```python
from build123d import *

# Parameters (mm, degrees)
F0_W     = 76.2
F0_H     = 63.5
F0_W_2   = 2.54
F0_H_2   = 27.94
F0_H_3   = 12.7
F1_DEPTH = 22.86
F2_W     = 76.2
F2_H     = 63.5
F3_DEPTH = 2.032
F4_R     = 1.27
F5_R     = 1


with BuildPart() as f1:
    # F0 (on Top) → F1 (new body)
    with BuildSketch(Plane.XY):
        with Locations((38.1, 31.75)):
            Rectangle(F0_W, F0_H)
        Polygon((2.54, 48.26), (2.54, 60.96), (73.66, 60.96), (73.66, 48.26), (73.66, 45.72), (73.66, 33.02), (73.66, 30.48), (73.66, 2.54), (41.4866666667, 2.54), (38.9466666667, 2.54), (22.0133333333, 2.54), (19.4733333333, 2.54), (2.54, 2.54), (2.54, 30.48), (2.54, 33.02), (2.54, 45.72), align=None, mode=Mode.SUBTRACT)
        Polygon((73.66, 48.26), (2.54, 48.26), (2.54, 45.72), (37.465, 45.72), (40.005, 45.72), (73.66, 45.72), align=None)
        Polygon((37.465, 33.02), (2.54, 33.02), (2.54, 30.48), (19.4733333333, 30.48), (22.0133333333, 30.48), (38.9466666667, 30.48), (41.4866666667, 30.48), (73.66, 30.48), (73.66, 33.02), (40.005, 33.02), align=None)
        with Locations((20.7433333333, 16.51)):
            Rectangle(F0_W_2, F0_H_2)
        with Locations((40.2166666667, 16.51)):
            Rectangle(F0_W_2, F0_H_2)
        with Locations((38.735, 39.37)):
            Rectangle(F0_W_2, F0_H_3)
    extrude(amount=F1_DEPTH)

    # F2 (on face) → F3 (join)
    with BuildSketch(Plane.XY.offset(22.86)):
        with Locations((38.1, 31.75)):
            Rectangle(F2_W, F2_H)
    extrude(amount=-F3_DEPTH)

    # F4
    f4_edges = [f1.edges().sort_by_distance(p)[0] for p in [
        (76.2, 31.75, 0),
        (38.1, 0, 0),
        (0, 31.75, 0),
        (38.1, 63.5, 0),
        (0, 63.5, 11.43),
        (76.2, 63.5, 11.43),
        (0, 0, 11.43),
        (76.2, 0, 11.43),
    ]]
    fillet(f4_edges, radius=F4_R)

    # F5
    f5_edges = [f1.edges().sort_by_distance(p)[0] for p in [
        (73.66, 60.96, 10.414),
        (73.66, 48.26, 10.414),
        (73.66, 33.02, 10.414),
        (73.66, 2.54, 10.414),
        (38.946667, 2.54, 10.414),
        (19.473333, 2.54, 10.414),
        (19.473333, 30.48, 10.414),
        (38.946667, 30.48, 10.414),
        (2.54, 30.48, 10.414),
        (2.54, 2.54, 10.414),
        (2.54, 45.72, 10.414),
        (2.54, 33.02, 10.414),
        (73.66, 45.72, 10.414),
        (41.486667, 30.48, 10.414),
        (41.486667, 2.54, 10.414),
        (2.54, 60.96, 10.414),
        (2.54, 48.26, 10.414),
        (73.66, 30.48, 10.414),
        (22.013333, 2.54, 10.414),
        (22.013333, 30.48, 10.414),
        (40.005, 33.02, 10.414),
        (40.005, 45.72, 10.414),
        (37.465, 45.72, 10.414),
        (37.465, 33.02, 10.414),
    ]]
    fillet(f5_edges, radius=F5_R)


solid = f1.part
```
Here's how the part is built. I have some questions about the finished solid (model axes, mm). A direction names the side the tool comes from. Round coordinates to 2 decimals unless told otherwise and drop trailing zeros. Loops run counter-clockwise (first coordinate to the right, second up) from the corner with the lowest first, then second, coordinate; pieces in that order, holes last. Notation, with made-up numbers: (-27.5, 8) -> (13.5, 8) arc R29 ccw to (13.5, 36) -> close; hole circle Ø8 at (84.5, 33). An arc over 180 degrees is marked (long way). Answer as CSV lines item,"result". Start each with the question number.
1. Imagine slicing it at D-D on y = 52.5. Write out the boundary of the cut face in (x, z).
2. If we mould it in two halves opening along Y, with no side actions, what happens to faces 1 (the face through (38, 0, 12)), 2 (the face through (20, 39, 20.828)), 3 (the face through (76.2, 31, 12)), 4 (the face through (11, 30.48, 10))? For each: pulls with the +Y half, pulls with the -Y half, needs draft (parallel to the pull), parting line crosses it, or undercut.
3. Imagine slicing it at B-B on x = 53.5. Write out the boundary of the cut face in (y, z), plus the area to 3 significant figures.
4. I'm going to push flat-ended pins straight in: P1, Ø10, axis at x = 21, y = 17.5, coming from the -Z side; P2, Ø4, axis at x = 49, y = 56.5, coming from the -Z side. Where does each tip first touch, or does it pass through?
5. Imagine slicing it at C-C on z = 10. State how many separate pieces and enclosed holes the cut face has, plus the area to 3 significant figures.
6. I need wall thicknesses on probe 1 along Y at (x, z) = (59, 17.5); probe 2 along X at (y, z) = (25.5, 10); probe 3 along X at (y, z) = (38.5, 8.5) (3 decimals). Which ranges of each line are inside material? Lowest first, please. Write a range as from..to.
7. For faces 5 (the face through (38, 32, 22.86)), 6 (the face through (57, 17, 20.828)), which set-ups out of +Z, -Z, +X, -X, +Y, -Y let a thin tool reach every point of the face, with its end or its side?
8. Imagine slicing it at A-A on y = 15.5. Write out the boundary of the cut face in (x, z).
Solution:
1,outline,"(0, 1.27) arc R1.27 ccw to (1.27, 0) -> (2.54, 0) -> (2.54, 20.83) -> (73.66, 20.83) -> (73.66, 0) -> (74.93, 0) arc R1.27 ccw to (76.2, 1.27) -> (76.2, 22.86) -> (0, 22.86) -> close"
2,face 1,"pulls with the -Y half"
2,face 2,"undercut"
2,face 3,"needs draft"
2,face 4,"undercut"
3,outline,"(0, 1.27) arc R1.27 ccw to (1.27, 0) -> (2.54, 0) -> (2.54, 20.83) -> (30.48, 20.83) -> (30.48, 0) -> (33.02, 0) -> (33.02, 20.83) -> (45.72, 20.83) -> (45.72, 0) -> (48.26, 0) -> (48.26, 20.83) -> (60.96, 20.83) -> (60.96, 0) -> (62.23, 0) arc R1.27 ccw to (63.5, 1.27) -> (63.5, 22.86) -> (0, 22.86) -> close"
3,area,"340 mm²"
4,P1,"z = 0"
4,P2,"z = 20.83"
5,separate pieces,"1"
5,enclosed holes,"6"
5,area,"1,220 mm²"
6,probe 1,"0..2.54, 30.48..33.02, 45.72..48.26, 60.96..63.5"
6,probe 2,"0..2.54, 19.47..22.01, 38.95..41.49, 73.66..76.2"
6,probe 3,"0..2.54, 37.465..40.005, 73.66..76.2"
7,face 5,"+Z, +X, -X, +Y, -Y"
7,face 6,"-Z"
8,outline,"(0, 1.27) arc R1.27 ccw to (1.27, 0) -> (2.54, 0) -> (2.54, 20.83) -> (19.47, 20.83) -> (19.47, 0) -> (22.01, 0) -> (22.01, 20.83) -> (38.95, 20.83) -> (38.95, 0) -> (41.49, 0) -> (41.49, 20.83) -> (73.66, 20.83) -> (73.66, 0) -> (74.93, 0) arc R1.27 ccw to (76.2, 1.27) -> (76.2, 22.86) -> (0, 22.86) -> close"
